Part model, mm, in its own coordinate system. Face numbers are marked on the shaded views. A direction names the side the tool comes from. Give positions to 0.01 mm unless a question says otherwise; leave off trailing zeros. Order: outer loops, then holes, each group sorted by start corner. A loop starts at its lowest first (then second) coordinate and runs counter-clockwise, first axis right, second up. Notation, with made-up numbers: M 73.5,4 L 121.5,4 A32 ccw 121.5,42 Z; hole C -21.5,-17.75 d3. An arc over 180 degrees is marked long. One line per question, with ' | ' between items.
```python
from build123d import *

# Parameters (mm, degrees)
ESQUISSE1_W                  = 22
ESQUISSE1_H                  = 12
BOSS_EXTRU_1_DEPTH           = 3
ESQUISSE3_R                  = 3
BOSS_EXTRU_3_DEPTH           = 3.5
ESQUISSE4_R                  = 1.25
ENL_V_MAT_EXTRU_1_DEPTH      = 28.789386463
BOSS_EXTRU_4_DEPTH           = 7.5
ENL_V_MAT_EXTRU_2_DEPTH      = 30.171904292
ENL_V_MAT_EXTRU_2_DEPTH_BACK = 30.171904292
ESQUISSE6_R                  = 3


with BuildPart() as part:
    # Esquisse1 → Boss.-Extru.1 (new body)
    with BuildSketch(Plane.XY):
        with BuildLine():
            Line((-17, -14), (-17, -18))
            ThreePointArc((-17, -18), (-14, -21), (-11, -18))
            Line((-11, -18), (-11, -14))
            Line((-11, -14), (11, -14))
            Line((11, -14), (11, -18))
            ThreePointArc((11, -18), (14, -21), (17, -18))
            Line((17, -18), (17, -14))
            Line((17, -14), (17, 10))
            ThreePointArc((17, 10), (16.121320344, 12.121320344), (14, 13))
            Line((14, 13), (-14, 13))
            ThreePointArc((-14, 13), (-16.121320344, 12.121320344), (-17, 10))
            Line((-17, 10), (-17, -14))
        make_face()
        with Locations((0, 2)):
            Rectangle(ESQUISSE1_W, ESQUISSE1_H, mode=Mode.SUBTRACT)
    extrude(amount=BOSS_EXTRU_1_DEPTH)

    # Esquisse3 → Boss.-Extru.3 (add)
    with BuildSketch(Plane.XY.offset(3)):
        with Locations((14, 10)):
            Circle(ESQUISSE3_R)
        with Locations(Location((-14, 10, 0), (0, 0, 180))):
            Circle(ESQUISSE3_R)
        with Locations((-14, -18)):
            Circle(ESQUISSE3_R)
        with Locations((14, -18)):
            Circle(ESQUISSE3_R)
    extrude(amount=BOSS_EXTRU_3_DEPTH)

    # Esquisse4 → Enlèv. mat.-Extru.1 (cut, through all)
    with BuildSketch(Plane.XY.offset(6.5)):
        with Locations((-14, 10)):
            Circle(ESQUISSE4_R)
        with Locations((14, 10)):
            Circle(ESQUISSE4_R)
        with Locations((-14, -18)):
            Circle(ESQUISSE4_R)
        with Locations((14, -18)):
            Circle(ESQUISSE4_R)
    extrude(amount=-ENL_V_MAT_EXTRU_1_DEPTH, mode=Mode.SUBTRACT)

    # Esquisse5 → Boss.-Extru.4 (add, symmetric)
    with BuildSketch(Plane(origin=(0, 0, 0), x_dir=(0, 0, -1), z_dir=(1, 0, 0))):
        with BuildLine():
            Line((6, -14), (0, -14))
            Line((0, -14), (0, -4))
            Line((0, -4), (6, -4))
            ThreePointArc((6, -4), (11, -9), (6, -14))
        make_face()
    extrude(amount=BOSS_EXTRU_4_DEPTH, both=True)

    # Esquisse6 → Enlèv. mat.-Extru.2 (cut, two sides: drawn at the far end of the back side and taken through both)
    with BuildSketch(Plane(origin=(0, 0, 0), x_dir=(0, 0, -1), z_dir=(1, 0, 0)).offset(-ENL_V_MAT_EXTRU_2_DEPTH_BACK)):
        with Locations(Location((6, -9, 0), (0, 0, 180))):
            Circle(ESQUISSE6_R)
    extrude(amount=ENL_V_MAT_EXTRU_2_DEPTH + ENL_V_MAT_EXTRU_2_DEPTH_BACK, mode=Mode.SUBTRACT)


solid = part.part
```
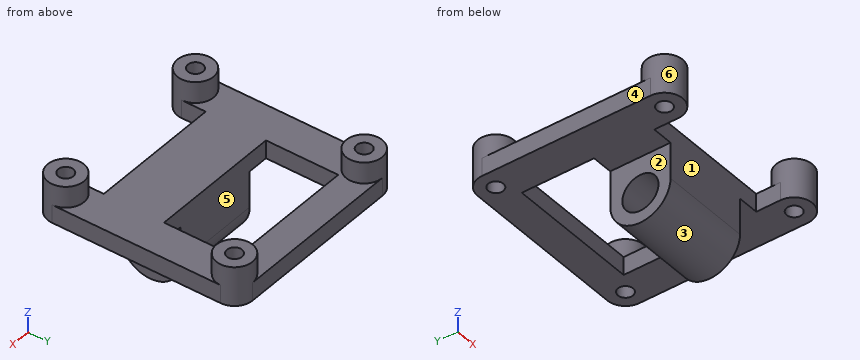
1. Probe L1, parallel to Y at x = -14, z = 4.75; L2, parallel to Y at x = 14, z = 1.5; L3, parallel to Y at x = -2.5, z = -6. List the from-to ranges inside material, lowest first. Write a range as from..to.
Worked out:
L1: y = -21..-19.25, -16.75..-15, 7..8.75, 11.25..13 | L2: y = -21..-19.25, -16.75..8.75, 11.25..13 | L3: y = -14..-12, -6..-4
2. Mould opens along X. For the marked faces 1, 2 and 3 say: released by +X, released by -X, zero draft, split by the parting line, or undercut.
Worked out:
face 1: undercut | face 2: released by -X | face 3: zero draft
3. Tool access for the marked faces 4, 5 and 6: list every direction of +Z, -Z, +X, -X, +Y, -Y with a clear straight run to the whole face (end or side of a thin tool).
Worked out:
face 4: +Z, -Z, -X, +Y, -Y | face 5: +Z, -Z | face 6: +Z
4. Slice it at C-C on z = -5. Give the cut face in (x, y), then the cut area to 3 significant figures.
Worked out:
outline: M -7.5,-14 L 7.5,-14 L 7.5,-11.83 L -7.5,-11.83 Z; M -7.5,-6.17 L 7.5,-6.17 L 7.5,-4 L -7.5,-4 Z | area: 65.1 mm2
5. Drop flat-ended pins along their axis: pin 1 (1.5 mm diameter, centred on x = 5, z = 2, fed in from -Y); pin 2 (2 mm diameter, centred on x = -2.5, z = -3, fed in from +Y); pin 3 (7 mm diameter, centred on y = -9, z = -6, fed in from -X); pin 4 (6 mm diameter, centred on y = -0.5, z = -8, fed in from +X). Give the stop position or say it passes through.
Worked out:
pin 1: stops at y = -14 | pin 2: stops at y = -4 | pin 3: stops at x = -7.5 | pin 4: passes through
6. Slice it at B-B on x = 3. Give the cut face in (y, z).
Worked out:
outline: M -14,-6 A5 ccw -4,-6 L -4,3 L -14,3 Z; M 8,0 L 13,0 L 13,3 L 8,3 Z; hole C -9,-6 d6
7. Slice it at A-A on y = 3. Give the cut face in (x, z).
Worked out:
outline: M -17,0 L -11,0 L -11,3 L -17,3 Z; M 11,0 L 17,0 L 17,3 L 11,3 Z
8. Slice it at D-D on y = -9. Give the cut face in (x, z), then the cut area to 3 significant figures.
Worked out:
outline: M -17,0 L -7.5,0 L -7.5,-3 L 7.5,-3 L 7.5,0 L 17,0 L 17,3 L -17,3 Z; M -7.5,-11 L 7.5,-11 L 7.5,-9 L -7.5,-9 Z | area: 177 mm2
